Model file for the job. Use its own axes, mm. A direction names the side the tool comes from. Coordinates: 2 decimals unless noted, no trailing zeros. Write each loop counter-clockwise with the first axis right and the second up, starting at its lowest first coordinate (ties: lowest second). Pieces come first, ordered by that corner, then holes.
Q1. Pin check, flat tips, straight feed: P1, Ø10, axis at x = 14, y = -6, coming from the -Z side; P2, Ø4, axis at x = 19.5, z = 12, coming from the -Y side; P3, Ø3.5, axis at x = 17, z = 18.5, coming from the +Y side. Stop position of each tip, or through.
Q2. Drill centre lines: probe 1 along Z at (x, y) = (12.5, 18.25); probe 2 along Y at (x, z) = (10.25, 15.5); probe 3 along Y at (x, z) = (1.5, 14). Where is each one in solid material? Low to high.
Q3. Band-saw the part on B-B, the plane x = 22.75. Write the cut outline in (y, z).
Q4. Pull direction Y, two halves, no side cores. Call faces 6 (the flat face through (12, -8.262, 19)), 7 (the flat face through (12, -10, 15.391)), 8 (the flat face through (5.684, 9.16, 30.646)): released by +Y, released by -Y, zero draft, split by the parting line, or undercut.
Q5. Which spindle directions (+Z, -Z, +X, -X, +Y, -Y) get a long thin tool onto all of the face, cutting with end or side? Do faces 1 (the flat face through (19.184, 9.16, 30.646)), 2 (the flat face through (12, 17, 4.741)), 3 (the cylindrical face through (24.285, 11.038, 12.273)), 4 (the cylindrical face through (0.715, 16.161, 4.041)), 5 (the cylindrical face through (10.02, 15.33, 0.47)). Say none if no direction does.
Q6. Band-saw the part on C-C, the plane x = 12.5. Write the cut outline in (y, z), plus the area to 3 significant figures.
from build123d import *

# Parameters (mm, degrees)
F0_W      = 10
F0_H      = 10.1
F1_DEPTH  = 25
F3_DEPTH  = 24.6375403377
F4_R      = 2.6
F5_DEPTH  = 33.001
F7_DEPTH  = 1
F9_DEPTH  = 1
F11_DEPTH = 1
F12_R     = 0.99999
F13_R     = 0.99999


# Not quite as in the source:
# - a fillet or chamfer is up to 0.001 mm smaller than in the source, because OpenCascade refuses the exact size


with BuildPart() as f1:
    # F0 (on Right) → F1 (new body)
    with BuildSketch(Plane.YZ):
        Polygon((8.7376843859, -5.3593200147), (3.235891927, -5.3593200147), (3.235891927, -8.3593200147), (8.7376843859, -8.3593200147), (11.7376843859, -8.3593200147), (11.7376843859, -5.3593200147), (11.7376843859, 4.7406799853), (11.7376843859, 20.9479271312), (2.9139854062, 22.7205907531), (-8.2623156141, 24.9658874581), (-8.2623156141, 21.9059462631), (-5.6975004546, 21.3906799853), (8.7376843859, 18.4906799853), align=None)
        Polygon((-8.2623156141, 15.3906799853), (-8.2623156141, 21.9059462631), (-8.2623156141, 24.9658874581), (-8.6975004546, 25.0533152293), (-11.2623156141, 25.5685815071), (-11.2623156141, 15.3906799853), (-8.6975004546, 15.3906799853), align=None)
        with Locations((16.7376843859, -0.3093200147)):
            Rectangle(F0_W, F0_H)
        Polygon((4.6866490281, 31.5442897327), (2.9139854062, 22.7205907531), (11.7376843859, 20.9479271312), (13.5103480077, 29.7716261109), align=None)
    extrude(amount=F1_DEPTH)

    # F2 (on face) → F3 (cut, through all)
    with BuildSketch(Plane(origin=(0, 7.2371941298, -1.4539379446), x_dir=(-1, 0, 0), z_dir=(0, 0.9804109977, -0.1969626246))):
        with BuildLine():
            ThreePointArc((-14.5, 28.8494632633), (-13.290569415, 24.9777550181), (-10, 27.3494632633))
            ThreePointArc((-10, 27.3494632633), (-10.1282917549, 28.1400326783), (-10.5, 28.8494632633))
            ThreePointArc((-10.5, 28.8494632633), (-12.5, 29.8494632633), (-14.5, 28.8494632633))
        make_face()
        with BuildLine():
            ThreePointArc((-14.5, 28.8494632633), (-12.5, 29.8494632633), (-10.5, 28.8494632633))
            Line((-10.5, 28.8494632633), (-10.5, 31.8494632633))
            Line((-10.5, 31.8494632633), (-12.5, 31.8494632633))
            Line((-12.5, 31.8494632633), (-14.5, 31.8494632633))
            Line((-14.5, 31.8494632633), (-14.5, 28.8494632633))
        make_face()
    extrude(amount=-F3_DEPTH, mode=Mode.SUBTRACT)

    # F4 (on face) → F5 (cut, through all)
    with BuildSketch(Plane(origin=(0, 21.7376843859, 0), x_dir=(-1, 0, 0), z_dir=(0, 1, 0))):
        with Locations((-12.5, -0.3093200147)):
            Circle(F4_R)
    extrude(amount=-F5_DEPTH, mode=Mode.SUBTRACT)

    # F6 (on face) → F7 (cut)
    with BuildSketch(Plane(origin=(0, 0, 0), x_dir=(0, -1, 0), z_dir=(-1, 0, 0))):
        Polygon((0.6576159399, 20.3781771837), (8.2623156141, 15.3906799853), (8.2623156141, 21.9059462631), align=None)
    extrude(amount=-F7_DEPTH, mode=Mode.SUBTRACT)

    # F8 (on face) → F9 (cut)
    with BuildSketch(Plane.YZ.offset(25)):
        Polygon((-11.2623156141, 15.3906799853), (-8.2623156141, 15.3906799853), (-8.2623156141, 16.3906799853), (-10.2623156141, 16.3906799853), (-10.2623156141, 24.3477030924), (3.6974337793, 21.5432171307), (5.4700974012, 30.3669161103), (12.3329743853, 28.9881777378), (10.7376843859, 21.0473825599), (10.7376843859, 3.7406799853), (20.7376843859, 3.7406799853), (20.7376843859, -4.3593200147), (10.7376843859, -4.3593200147), (10.7376843859, -7.3593200147), (4.235891927, -7.3593200147), (4.235891927, -5.3593200147), (3.235891927, -5.3593200147), (3.235891927, -8.3593200147), (11.7376843859, -8.3593200147), (11.7376843859, -5.3593200147), (21.7376843859, -5.3593200147), (21.7376843859, 4.7406799853), (11.7376843859, 4.7406799853), (11.7376843859, 20.9479271312), (13.5103480077, 29.7716261109), (4.6866490281, 31.5442897327), (2.9139854062, 22.7205907531), (-11.2623156141, 25.5685815071), align=None)
    extrude(amount=-F9_DEPTH, mode=Mode.SUBTRACT)

    # F10 (on face) → F11 (cut)
    with BuildSketch(Plane(origin=(0, 0, 0), x_dir=(0, -1, 0), z_dir=(-1, 0, 0))):
        Polygon((8.2623156141, 16.3906799853), (8.2623156141, 15.3906799853), (11.2623156141, 15.3906799853), (11.2623156141, 25.5685815071), (-2.9139854062, 22.7205907531), (-4.6866490281, 31.5442897327), (-13.5103480077, 29.7716261109), (-11.7376843859, 20.9479271312), (-11.7376843859, 4.7406799853), (-21.7376843859, 4.7406799853), (-21.7376843859, -5.3593200147), (-11.7376843859, -5.3593200147), (-11.7376843859, -8.3593200147), (-3.235891927, -8.3593200147), (-3.235891927, -5.3593200147), (-4.235891927, -5.3593200147), (-4.235891927, -7.3593200147), (-10.7376843859, -7.3593200147), (-10.7376843859, -4.3593200147), (-20.7376843859, -4.3593200147), (-20.7376843859, 3.7406799853), (-10.7376843859, 3.7406799853), (-10.7376843859, 21.0473825599), (-12.3329743853, 28.9881777378), (-5.4700974012, 30.3669161103), (-3.6974337793, 21.5432171307), (10.2623156141, 24.3477030924), (10.2623156141, 16.3906799853), align=None)
    extrude(amount=-F11_DEPTH, mode=Mode.SUBTRACT)

    # F12 (radius 1 in the source; OpenCascade refuses exactly that, so slightly less here)
    f12_edges = [f1.edges().sort_by_distance(p)[0] for p in [
        (24, 4.235892, -6.35932),
        (24, 7.486788, -7.35932),
        (24, 15.737684, -4.35932),
        (24, 10.737684, -5.85932),
        (24, 20.737684, -0.30932),
        (24, 10.737684, 12.394031),
        (24, 15.737684, 3.74068),
        (24, 11.535329, 25.01778),
        (24, 8.901536, 29.677547),
        (24, -3.282441, 22.94546),
        (24, 4.583766, 25.955067),
        (24, -10.262316, 20.369192),
        (24, -9.262316, 16.39068),
    ]]
    fillet(f12_edges, radius=F12_R)

    # F13 (radius 1 in the source; OpenCascade refuses exactly that, so slightly less here)
    f13_edges = [f1.edges().sort_by_distance(p)[0] for p in [
        (1, 4.235892, -6.35932),
        (1, 7.486788, -7.35932),
        (1, 15.737684, -4.35932),
        (1, 10.737684, -5.85932),
        (1, 20.737684, -0.30932),
        (1, 10.737684, 12.394031),
        (1, 15.737684, 3.74068),
        (1, 11.535329, 25.01778),
        (1, 8.901536, 29.677547),
        (1, -3.282441, 22.94546),
        (1, 4.583766, 25.955067),
        (1, -10.262316, 20.369192),
        (1, -9.262316, 16.39068),
    ]]
    fillet(f13_edges, radius=F13_R)


solid = f1.part
Answer sheet:
1. P1: stops at z = 15.39
1. P2: stops at y = 8.74
1. P3: stops at y = 11.74
2. probe 1: z = -5.36 to -2.91, 2.29 to 4.74
2. probe 2: y = -11.26 to -8.26, 8.74 to 11.74
2. probe 3: y = 8.74 to 11.74
3. outline: (-11.26, 15.39) - (-8.26, 15.39) - (-8.26, 21.91) - (8.74, 18.49) - (8.74, -5.36) - (3.24, -5.36) - (3.24, -8.36) - (11.74, -8.36) - (11.74, -5.36) - (21.74, -5.36) - (21.74, 4.74) - (11.74, 4.74) - (11.74, 20.95) - (13.51, 29.77) - (4.69, 31.54) - (2.91, 22.72) - (-11.26, 25.57) - close
4. face 6: undercut
4. face 7: zero draft
4. face 8: released by +Y
5. face 1: +Z, +X, -X, +Y
5. face 2: +X, -X, +Y
5. face 3: +X, +Y
5. face 4: -X, +Y
5. face 5: +Y, -Y
6. outline: (-11.26, 15.39) - (-8.26, 15.39) - (-8.26, 21.91) - (8.74, 18.49) - (8.74, 2.29) - (21.74, 2.29) - (21.74, 4.74) - (11.74, 4.74) - (11.74, 20.95) - (12.13, 22.91) - (3.31, 24.68) - (2.91, 22.72) - (-11.26, 25.57) - close; (3.24, -8.36) - (11.74, -8.36) - (11.74, -5.36) - (21.74, -5.36) - (21.74, -2.91) - (8.74, -2.91) - (8.74, -5.36) - (3.24, -5.36) - close
6. area: 238 mm2
